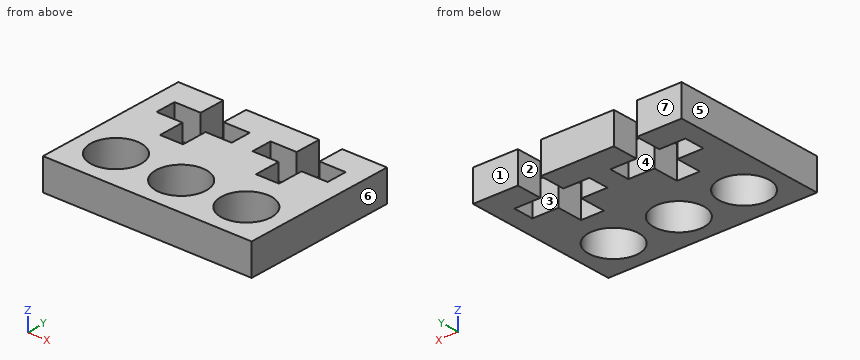
from build123d import *

# Parameters (mm, degrees)
SKETCH1_R           = 2.4
BOSS_EXTRUDE1_DEPTH = 3


with BuildPart() as part:
    # Sketch1 → Boss-Extrude1 (new body)
    with BuildSketch(Plane.XY):
        Polygon((-10, -7.5), (10, -7.5), (10, 7.5), (5.7, 7.5), (5.7, 5), (8.2, 5), (8.2, 3), (5.7, 3), (5.7, 0.5), (3.5, 0.5), (3.5, 3), (1, 3), (1, 5), (3.5, 5), (3.5, 7.5), (-3.5, 7.5), (-3.5, 5), (-1, 5), (-1, 3), (-3.5, 3), (-3.5, 0.5), (-5.7, 0.5), (-5.7, 3), (-8.2, 3), (-8.2, 5), (-5.7, 5), (-5.7, 7.5), (-10, 7.5), align=None)
        with Locations((0, -3.75)):
            Circle(SKETCH1_R, mode=Mode.SUBTRACT)
        with Locations((-6.25, -3.75)):
            Circle(SKETCH1_R, mode=Mode.SUBTRACT)
        with Locations((6.25, -3.75)):
            Circle(SKETCH1_R, mode=Mode.SUBTRACT)
    extrude(amount=BOSS_EXTRUDE1_DEPTH)


solid = part.part
Verification items for the finished model (mm, model axes). Face numbers are marked on the shaded views. A direction names the side the tool comes from. Coordinates: 2 decimals unless noted, no trailing zeros. Write each loop counter-clockwise with the first axis right and the second up, starting at its lowest first coordinate (ties: lowest second). Pieces come first, ordered by that corner, then holes. Notation, with made-up numbers: (42.25, 54.25) - (94.25, 54.25) arc R24 ccw to (94.25, 76.25) - close; hole circle Ø10 at (-21.5, -22.5). An arc over 180 degrees is marked (long way). Answer as a JSON object with one key per item and string values.
(1) Gauge pin test, flat ends, axial feed: pin 1 Ø3 at (x, y) = (0, -3.75) entering from -Z; pin 2 Ø0.7 at (x, z) = (5, 1.5) entering from +Y. Record the tip position at first contact, or that the pin passes through.
Report:
{"pin 1": "through", "pin 2": "y = 0.5"}
(2) Cross-section at D-D on x = -6. Record the cut outline in (y, z).
Report:
{"outline": "(-7.5, 0) - (-6.14, 0) - (-6.14, 3) - (-7.5, 3) - close; (-1.36, 0) - (3, 0) - (3, 3) - (-1.36, 3) - close; (5, 0) - (7.5, 0) - (7.5, 3) - (5, 3) - close"}
(3) Thickness scan on line 1 along Y through (x, z) = (-6.25, 2.45); line 2 along X through (y, z) = (4.25, 2.8); line 3 along Y through (x, z) = (2.5, 0.4). Record the ranges inside material, lowest first.
Report:
{"line 1": "-7.5 to -6.15, -1.35 to 3, 5 to 7.5", "line 2": "-10 to -8.2, -1 to 1, 8.2 to 10", "line 3": "-7.5 to 3, 5 to 7.5"}
(4) Mould release check, pull along X, two halves, no side actions. Record for the marked faces 4, 5, 6 and 7: pulls with the +X half, pulls with the -X half, needs draft (parallel to the pull), parting line crosses it, or undercut.
Report:
{"face 4": "undercut", "face 5": "pulls with the -X half", "face 6": "pulls with the +X half", "face 7": "needs draft"}
(5) Cross-section at A-A on y = 6.25. Record the cut outline in (x, z), plus the area to 3 significant figures.
Report:
{"outline": "(-10, 0) - (-5.7, 0) - (-5.7, 3) - (-10, 3) - close; (-3.5, 0) - (3.5, 0) - (3.5, 3) - (-3.5, 3) - close; (5.7, 0) - (10, 0) - (10, 3) - (5.7, 3) - close", "area": "46.8 mm^2"}
(6) Tool access check on the marked faces 1, 2 and 3. Record the directions out of +Z, -Z, +X, -X, +Y, -Y that give a thin tool (end or side, any length) a straight path to the whole face; none if there is none.
Report:
{"face 1": "+Z, -Z, +X, -X, +Y", "face 2": "+Z, -Z, +Y", "face 3": "+Z, -Z"}
(7) Cross-section at B-B on z = 1.3. Give the number of separate pieces and of enclosed holes in the cut face, plus the area to 3 significant figures.
Report:
{"separate pieces": "1", "enclosed holes": "3", "area": "195 mm^2"}
(8) Cross-section at C-C on y = -3.75. Record the cut outline in (x, z), plus the area to 3 significant figures.
Report:
{"outline": "(-10, 0) - (-8.65, 0) - (-8.65, 3) - (-10, 3) - close; (-3.85, 0) - (-2.4, 0) - (-2.4, 3) - (-3.85, 3) - close; (2.4, 0) - (3.85, 0) - (3.85, 3) - (2.4, 3) - close; (8.65, 0) - (10, 0) - (10, 3) - (8.65, 3) - close", "area": "16.8 mm^2"}
